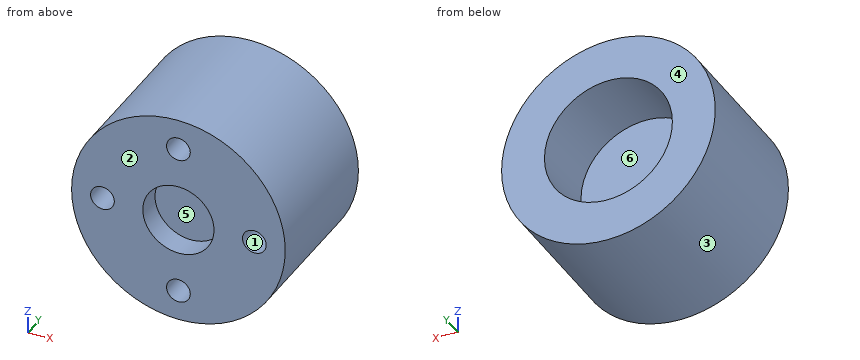
```python
from build123d import *

# Parameters (mm, degrees)
F0_R     = 22.5
F1_DEPTH = 30
F2_R     = 7.5
F3_DEPTH = 5
F4_R     = 2.5
F5_DEPTH = 10
F6_R     = 13.475
F7_DEPTH = 15


with BuildPart() as f1:
    # F0 (on Front) → F1 (new body)
    with BuildSketch(Plane.XZ):
        Circle(F0_R)
    extrude(amount=F1_DEPTH)

    # F2 (on face) → F3 (cut)
    with BuildSketch(Plane.XZ.offset(30)):
        Circle(F2_R)
    extrude(amount=-F3_DEPTH, mode=Mode.SUBTRACT)

    # F4 (on face) → F5 (cut)
    with BuildSketch(Plane.XZ.offset(30)):
        with Locations((-16, 0)):
            Circle(F4_R)
        with Locations((0, 16)):
            Circle(F4_R)
        with Locations((16, 0)):
            Circle(F4_R)
        with Locations((0, -16)):
            Circle(F4_R)
    extrude(amount=-F5_DEPTH, mode=Mode.SUBTRACT)

    # F6 (on face) → F7 (cut)
    with BuildSketch(Plane(origin=(0, 0, 0), x_dir=(-1, 0, 0), z_dir=(0, 1, 0))):
        Circle(F6_R)
    extrude(amount=-F7_DEPTH, mode=Mode.SUBTRACT)


solid = f1.part
```
Source: CAD feature listing. Evaluate the final solid. Frame: model axes, mm. Face numbers are marked on the shaded views. A direction names the side the tool comes from. Give positions to 0.01 mm unless a question says otherwise; leave off trailing zeros. Write each loop counter-clockwise with the first axis right and the second up, starting at its lowest first coordinate (ties: lowest second). Pieces come first, ordered by that corner, then holes.
1. First-contact query: pin 1 (12 mm diameter, centred on y = -19, z = -16.5, fed in from +X); pin 2 (12 mm diameter, centred on y = -16, z = 6, fed in from -X); pin 3 (4.5 mm diameter, centred on x = -16, z = 0, fed in from -Y); pin 4 (7.5 mm diameter, centred on x = -2.5, z = -1, fed in from -Y). Flat tips, straight axial feed; report the tip coordinate or a pass-through.
2. Section query D-D (y = -22.5). Return the cut outline in (x, z), then the cut area to 3 significant figures.
3. Section query B-B (z = 0). Return the cut outline in (x, y) (3 decimals).
4. Section query C-C (x = 0). Return the cut outline in (y, z) (3 decimals), then the cut area to 3 significant figures.
5. Section query A-A (y = -27). Return the cut outline in (x, z).
6. Access query for the marked faces 4, 5 and 6. Directions: +Z, -Z, +X, -X, +Y, -Y. A direction counts if a zero-diameter tool reaches every point of the face in a straight line with its end or side. Return the directions, or none.
7. Pull-direction query (Z, two-part tool) for the marked faces 1, 2 and 3; classes: +Z half, -Z half, draft (parallel to the pull), parting line (faces both ways), or undercut.
8. Material intervals for line 1 along Z through (x, y) = (0, -7) (3 decimals); line 2 along X through (y, z) = (-25.75, -1.5); line 3 along X through (y, z) = (-19.25, -0.5), sorted ascending.
Output values:
1. pin 1: stops at x = 19.9
1. pin 2: stops at x = -22.5
1. pin 3: stops at y = -20
1. pin 4: stops at y = -25
2. outline: circle Ø45 at (0, 0); hole circle Ø5 at (-16, 0); hole circle Ø5 at (0, -16); hole circle Ø5 at (0, 16); hole circle Ø5 at (16, 0)
2. area: 1,510 mm2
3. outline: (-22.5, -30) - (-18.5, -30) - (-18.5, -20) - (-13.5, -20) - (-13.5, -30) - (-7.5, -30) - (-7.5, -25) - (7.5, -25) - (7.5, -30) - (13.5, -30) - (13.5, -20) - (18.5, -20) - (18.5, -30) - (22.5, -30) - (22.5, 0) - (13.475, 0) - (13.475, -15) - (-13.475, -15) - (-13.475, 0) - (-22.5, 0) - close
4. outline: (-30, -22.5) - (0, -22.5) - (0, -13.475) - (-15, -13.475) - (-15, 13.475) - (0, 13.475) - (0, 22.5) - (-30, 22.5) - (-30, 18.5) - (-20, 18.5) - (-20, 13.5) - (-30, 13.5) - (-30, 7.5) - (-25, 7.5) - (-25, -7.5) - (-30, -7.5) - (-30, -13.5) - (-20, -13.5) - (-20, -18.5) - (-30, -18.5) - close
4. area: 771 mm2
5. outline: circle Ø45 at (0, 0); hole circle Ø5 at (-16, 0); hole circle Ø15 at (0, 0); hole circle Ø5 at (0, -16); hole circle Ø5 at (0, 16); hole circle Ø5 at (16, 0)
6. face 4: +Z, -Z, +X, -X, +Y
6. face 5: -Y
6. face 6: +Y
7. face 1: undercut
7. face 2: draft
7. face 3: parting line
8. line 1: z = -22.5 to -13.475, 13.475 to 22.5
8. line 2: x = -22.45 to -18, -14 to -7.35, 7.35 to 14, 18 to 22.45
8. line 3: x = -22.49 to 22.49
